The model under review builds one solid part; all positions refer to its coordinate system, in mm. A direction names the side the tool comes from. Round coordinates to 2 decimals unless told otherwise and drop trailing zeros. Order: outer loops, then holes, each group sorted by start corner. A loop starts at its lowest first (then second) coordinate and runs counter-clockwise, first axis right, second up. Notation, with made-up numbers: M 75,87.25 L 113,87.25 A24 ccw 113,111.25 Z; hole C 69.25,22.5 d6. An arc over 180 degrees is marked long. Answer as a JSON object with one key per item and string values. Group by question number.
1. Add section B-B on z = 9.5. State the section outline as (x, y) points, and give its area (3 significant figures).
2. To check wall thickness, follow probe 1 along Y at (x, z) = (55.5, -6) (3 decimals); probe 2 along Y at (x, z) = (64, -9); probe 3 along Y at (x, z) = (67.5, 3). State the ranges of each line that lie inside material, in increasing order. Write a range as [from, to].
3. Clearance check with flat-ended pins moving along their axes: P1, Ø6, axis at x = 74.5, z = -16.5, coming from the -Y side; P2, Ø4, axis at x = 57, z = -5.5, coming from the +Y side (3 decimals); P3, Ø1.3, axis at y = 73.5, z = 6.5, coming from the +X side; P4, Ø4, axis at y = 81, z = -1.5, coming from the -X side. State where each tip first meets the part, or that it passes through.
4. Add section D-D on z = -7.5. State the section outline as (x, y) points (3 decimals), and give its area (3 significant figures).
5. Add section A-A on y = 59. State the section outline as (x, z) points (3 decimals).
6. Mouldability with a two-part tool opening along Y and no side actions: class faces 5 (the face through (57, -3.175, -7)), 6 (the face through (57.11, -2.9, -0.36)), 7 (the face through (57, -1, -28.575)) as released by +Y, released by -Y, zero draft, split by the parting line, or undercut.
7. Machinability: for faces 1 (the face through (57.114, -2.817, -13.257)), 2 (the face through (55.021, 50, 3)), 3 (the face through (55.021, 26, 9)), 4 (the face through (59.69, -4, -7)), which of the approach directions +Z, -Z, +X, -X, +Y, -Y give a long, thin tool a straight path to every point of the face, cutting with its end or side? Answer none if there is none.
8. Add section C-C on x = 67. State the section outline as (y, z) points (3 decimals), and give its area (3 significant figures).
```python
from build123d import *

# Parameters (mm, degrees)
SKETCH1_W             = 76.2
SKETCH1_H             = 114.3
BOSS_EXTRUDE1_DEPTH   = 2.54
SKETCH2_W             = 20.32
SKETCH2_H             = 41.91
CUT_EXTRUDE1_DEPTH    = 138.394983897
SKETCH3_W             = 76.2
SKETCH3_H             = 6.35
BOSS_EXTRUDE2_DEPTH   = 28.575
SKETCH4_W             = 76.2
SKETCH4_H             = 9.525
BOSS_EXTRUDE3_DEPTH   = 3.175
F_6_CLEARANCE_HOLE1_D = 4.3053
SKETCH9_W             = 76.2
SKETCH9_H             = 114.3
SKETCH9_W_2           = 20.32
SKETCH9_H_2           = 41.91
BOSS_EXTRUDE4_DEPTH   = 3.175
SKETCH10_W            = 38.1
SKETCH10_H            = 133.35
CUT_EXTRUDE3_DEPTH    = 150.381641191
SKETCH11_W            = 20.32
SKETCH11_H            = 6.985
BOSS_EXTRUDE5_DEPTH   = 6.35
F_6_32_TAPPED_HOLE1_D = 2.7051
SKETCH15_W            = 6.35
SKETCH15_H            = 2.54
CUT_EXTRUDE4_DEPTH    = 151.965824692
SKETCH16_W            = 20.32
SKETCH16_H            = 43.688
CUT_EXTRUDE5_DEPTH    = 151.965824692
SKETCH17_W            = 6.35
SKETCH17_H            = 81.28
BOSS_EXTRUDE6_DEPTH   = 5.715
FILLET1_START         = -28.575
FILLET1_DEPTH         = 35.575
FILLET1_2_DEPTH       = 5.715
BOSS_EXTRUDE7_START   = -19.05
BOSS_EXTRUDE7_DEPTH   = 2.54


with BuildPart() as part:
    # Sketch1 → Boss-Extrude1 (new body)
    with BuildSketch(Plane.XY):
        with Locations((38.1, 57.15)):
            Rectangle(SKETCH1_W, SKETCH1_H)
    extrude(amount=BOSS_EXTRUDE1_DEPTH)

    # Sketch2 → Cut-Extrude1 (cut, through all)
    with BuildSketch(Plane.XY.offset(2.54)):
        with Locations((65.18148, 50.70348)):
            Rectangle(SKETCH2_W, SKETCH2_H)
    extrude(amount=-CUT_EXTRUDE1_DEPTH, mode=Mode.SUBTRACT)

    # Sketch3 → Boss-Extrude2 (add)
    with BuildSketch(Plane(origin=(0, 0, 0), x_dir=(-1, 0, 0), z_dir=(0, 0, -1))):
        with Locations((-38.1, 111.125)):
            Rectangle(SKETCH3_W, SKETCH3_H)
        with Locations((-38.1, 3.175)):
            Rectangle(SKETCH3_W, SKETCH3_H)
    extrude(amount=BOSS_EXTRUDE2_DEPTH)

    # Sketch4 → Boss-Extrude3 (add)
    with BuildSketch(Plane(origin=(0, 0, -28.575), x_dir=(-1, 0, 0), z_dir=(0, 0, -1))):
        with Locations((-38.1, 119.0625)):
            Rectangle(SKETCH4_W, SKETCH4_H)
        with Locations((-38.1, -4.7625)):
            Rectangle(SKETCH4_W, SKETCH4_H)
    extrude(amount=-BOSS_EXTRUDE3_DEPTH)

    # #6 Clearance Hole1 (through all)
    with Locations(Plane.XY.offset(-25.4)):
        with Locations((9.525, 118.745), (9.525, -4.445), (22.225, -4.445), (34.925, -4.445), (47.625, -4.445), (60.325, -4.445), (22.225, 118.745), (73.025, -4.445), (34.925, 118.745), (47.625, 118.745), (60.325, 118.745), (73.025, 118.745)):
            Hole(F_6_CLEARANCE_HOLE1_D / 2)

    # Sketch9 → Boss-Extrude4 (add)
    with BuildSketch(Plane.XY.offset(2.54)):
        with Locations((38.1, 57.15)):
            Rectangle(SKETCH9_W, SKETCH9_H)
        with Locations((65.18148, 50.70348)):
            Rectangle(SKETCH9_W_2, SKETCH9_H_2, mode=Mode.SUBTRACT)
    extrude(amount=BOSS_EXTRUDE4_DEPTH)

    # Sketch10 → Cut-Extrude3 (cut, through all)
    with BuildSketch(Plane.XY.offset(5.715)):
        with Locations((19.05, 57.15)):
            Rectangle(SKETCH10_W, SKETCH10_H)
    extrude(amount=-CUT_EXTRUDE3_DEPTH, mode=Mode.SUBTRACT)

    # Sketch11 → Boss-Extrude5 (add)
    with BuildSketch(Plane.XY.offset(5.715)):
        with Locations((65.18148, 75.15098)):
            Rectangle(SKETCH11_W, SKETCH11_H)
        with Locations((65.18148, 26.25598)):
            Rectangle(SKETCH11_W, SKETCH11_H)
    extrude(amount=BOSS_EXTRUDE5_DEPTH)

    # #6-32 Tapped Hole1 (through all)
    with Locations(Plane(origin=(0, 0, 0), x_dir=(-1, 0, 0), z_dir=(0, 0, -1))):
        with Locations((-70.18147, 75.45324), (-60.18149, 75.45324), (-60.18149, 25.95372), (-70.18147, 25.95372)):
            Hole(F_6_32_TAPPED_HOLE1_D / 2)

    # Sketch15 → Cut-Extrude4 (cut, through all)
    with BuildSketch(Plane.XY.offset(12.065)):
        with Locations((65.18148, 72.92848)):
            Rectangle(SKETCH15_W, SKETCH15_H)
    extrude(amount=-CUT_EXTRUDE4_DEPTH, mode=Mode.SUBTRACT)

    # Sketch16 → Cut-Extrude5 (cut, through all)
    with BuildSketch(Plane.XY.offset(12.065)):
        with Locations((65.18148, 50.70348)):
            Rectangle(SKETCH16_W, SKETCH16_H)
    extrude(amount=-CUT_EXTRUDE5_DEPTH, mode=Mode.SUBTRACT)

    # Sketch17 → Boss-Extrude6 (add)
    with BuildSketch(Plane.XY.offset(5.715)):
        with Locations((79.375, 50.70348)):
            Rectangle(SKETCH17_W, SKETCH17_H)
    extrude(amount=-BOSS_EXTRUDE6_DEPTH)

    # Fillet1: read off the stored shape, not the designer's step
    # Fillet1 outline → Fillet1 (cut)
    with BuildSketch(Plane.XY.offset(FILLET1_START)):
        with BuildLine():
            ThreePointArc((79.375, 91.34348), (81.62006403, 90.41354403), (82.55, 88.16848))
            Line((82.55, 88.16848), (82.55, 91.34348))
            Line((82.55, 91.34348), (79.375, 91.34348))
        make_face()
        with BuildLine():
            ThreePointArc((82.55, 13.23848), (81.62006403, 10.99341597), (79.375, 10.06348))
            Line((79.375, 10.06348), (82.55, 10.06348))
            Line((82.55, 10.06348), (82.55, 13.23848))
        make_face()
    extrude(amount=FILLET1_DEPTH, mode=Mode.SUBTRACT)

    # Fillet1 2 outline → Fillet1 2 (add)
    with BuildSketch(Plane.XY):
        with BuildLine():
            Line((76.2, 91.34348), (79.375, 91.34348))
            ThreePointArc((79.375, 91.34348), (77.12993597, 92.27341597), (76.2, 94.51848))
            Line((76.2, 94.51848), (76.2, 91.34348))
        make_face()
        with BuildLine():
            ThreePointArc((76.2, 6.88848), (77.12993597, 9.13354403), (79.375, 10.06348))
            Line((79.375, 10.06348), (76.2, 10.06348))
            Line((76.2, 10.06348), (76.2, 6.88848))
        make_face()
    extrude(amount=FILLET1_2_DEPTH)

    # Sketch18 → Boss-Extrude7 (add, symmetric)
    with BuildSketch(Plane.ZY.offset(-38.1).offset(BOSS_EXTRUDE7_START)):
        Polygon((-16.074204897, 114.3), (-10.359204897, 120.015), (-3.175, 120.015), (2.54, 114.3), (-1.052102448, 114.3), (-4.227102448, 117.475), (-9.307102448, 117.475), (-12.482102448, 114.3), align=None)
    boss_extrude7 = extrude(amount=BOSS_EXTRUDE7_DEPTH, both=True)

    # Mirror1: Boss-Extrude7 across plane
    add(boss_extrude7.mirror(Plane.ZX.offset(57.15)))


solid = part.part
```
Recorded:
{
 "1": {"outline": "M 55.02,22.76 L 75.34,22.76 L 75.34,28.86 L 55.02,28.86 Z; M 55.02,72.55 L 62.01,72.55 L 62.01,74.2 L 68.36,74.2 L 68.36,72.55 L 75.34,72.55 L 75.34,78.64 L 55.02,78.64 Z; hole C 60.18,25.95 d2.71; hole C 60.18,75.45 d2.71; hole C 70.18,25.95 d2.71; hole C 70.18,75.45 d2.71", "area": "214 mm²"},
 "2": {"probe 1": "y = [-5.715, -3.175], [0, 6.35], [107.95, 114.3], [117.475, 120.015]", "probe 2": "y = [0, 6.35], [107.95, 114.3]", "probe 3": "y = [0, 28.86], [74.2, 114.3]"},
 "3": {"P1": "stops at y = 0", "P2": "stops at y = 120.015", "P3": "stops at x = 75.34", "P4": "stops at x = 38.1"},
 "4": {"outline": "M 38.1,0 L 76.2,0 L 76.2,6.35 L 38.1,6.35 Z; M 38.1,107.95 L 76.2,107.95 L 76.2,114.3 L 38.1,114.3 Z; M 54.61,-5.715 L 59.69,-5.715 L 59.69,-3.175 L 54.61,-3.175 Z; M 54.61,117.475 L 59.69,117.475 L 59.69,120.015 L 54.61,120.015 Z", "area": "510 mm²"},
 "5": {"outline": "M 38.1,0 L 55.021,0 L 55.021,5.715 L 38.1,5.715 Z; M 75.341,0 L 82.55,0 L 82.55,5.715 L 75.341,5.715 Z"},
 "6": {"face 5": "undercut", "face 6": "released by -Y", "face 7": "zero draft"},
 "7": {"face 1": "+X, -X, -Y", "face 2": "+Z, -Z", "face 3": "+Z, -X, +Y, -Y", "face 4": "+Z, +X, -Y"},
 "8": {"outline": "M -9.525,-28.575 L 6.35,-28.575 L 6.35,0 L 28.859,0 L 28.859,12.065 L 22.763,12.065 L 22.763,5.715 L 0,5.715 L 0,-25.4 L -9.525,-25.4 Z; M 74.198,0 L 107.95,0 L 107.95,-28.575 L 123.825,-28.575 L 123.825,-25.4 L 114.3,-25.4 L 114.3,5.715 L 78.643,5.715 L 78.643,12.065 L 74.198,12.065 Z", "area": "884 mm²"}
}
